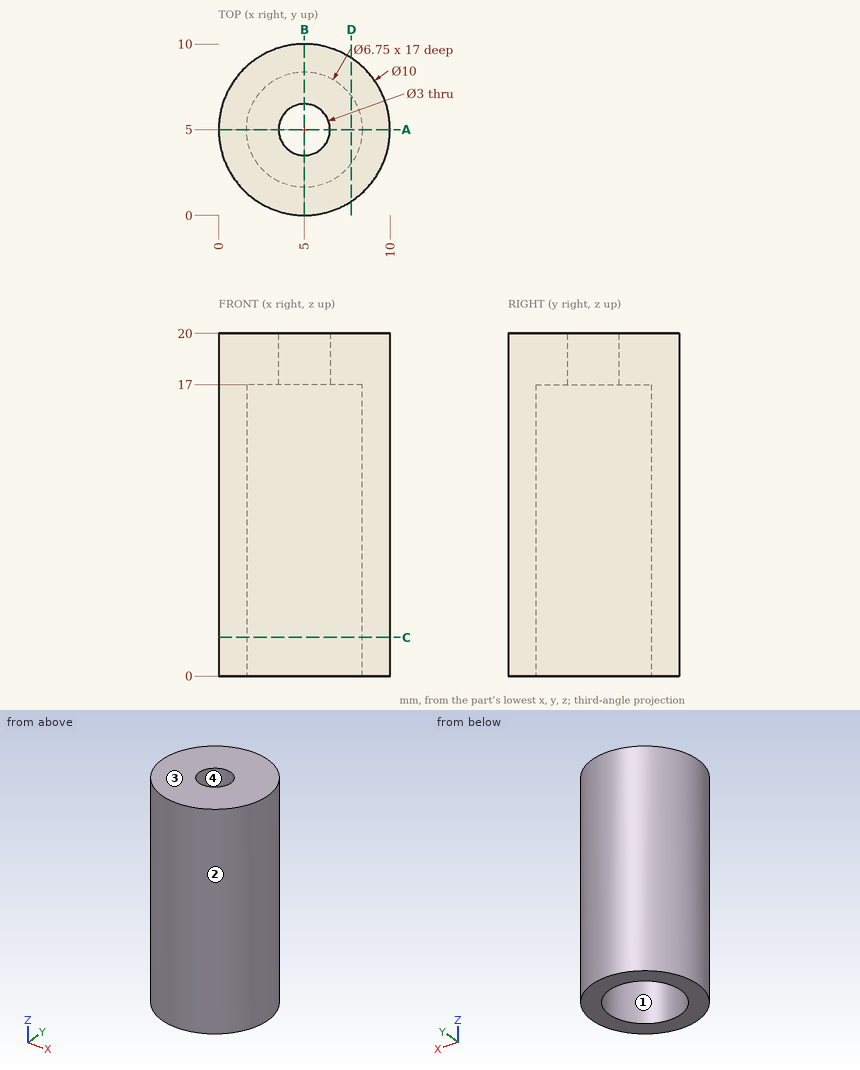
Check sheet for the drawn part. Datum: minimum x, y, z corner. Units: mm. Coordinates: 2 decimals unless noted, no trailing zeros. Loops run counter-clockwise (first coordinate to the right, second up) from the corner with the lowest first, then second, coordinate; pieces in that order, holes last. Notation, with made-up numbers: M -7,5.5 L 44,5.5 A12 cw 44,19.5 Z; hole C 17.25,28.5 d2. An arc over 180 degrees is marked long. Answer as a JSON object with one key per item and string values.
1. Sectioned sample at C-C on z = 2.25. Record the cut outline in (x, y) (3 decimals).
Outcome:
{"outline": "C 5,5 d10; hole C 5,5 d6.75"}
2. Scan lines: L1, parallel to Y at x = 5, z = 18.9; L2, parallel to Y at x = 5, z = 9 (3 decimals); L3, parallel to Z at x = 7, y = 5.75. Record each from-to range of solid material in increasing order. Write a range as from..to.
Outcome:
{"L1": "0..3.5, 6.5..10", "L2": "0..1.625, 8.375..10", "L3": "17..20"}
3. Sectioned sample at A-A on y = 5. Record the cut outline in (x, z) (3 decimals).
Outcome:
{"outline": "M 0,0 L 1.625,0 L 1.625,17 L 3.5,17 L 3.5,20 L 0,20 Z; M 6.5,17 L 8.375,17 L 8.375,0 L 10,0 L 10,20 L 6.5,20 Z"}
4. Sectioned sample at D-D on x = 7.75. Record the cut outline in (y, z).
Outcome:
{"outline": "M 0.82,0 L 3.04,0 L 3.04,17 L 6.96,17 L 6.96,0 L 9.18,0 L 9.18,20 L 0.82,20 Z"}
5. Release check for a two-part mould opening along X. For the marked faces 1, 2, 3 and 4 record: pulls with the +X half, pulls with the -X half, needs draft (parallel to the pull), parting line crosses it, or undercut.
Outcome:
{"face 1": "undercut", "face 2": "parting line crosses it", "face 3": "needs draft", "face 4": "undercut"}
6. Depth check by flat-ended pin: P1, Ø3, axis at x = 5.5, y = 5, coming from the -Z side. Enter the tip coordinate at first touch or a pass-through.
Outcome:
{"P1": "z = 17"}
